Here's how the part is built. I have some questions about the finished solid (model axes, mm). A direction names the side the tool comes from. Give positions to 0.01 mm unless a question says otherwise; leave off trailing zeros. Loops run counter-clockwise (first coordinate to the right, second up) from the corner with the lowest first, then second, coordinate; pieces in that order, holes last.
Q1. I need wall thicknesses on probe 1 along Y at (x, z) = (26.5, 4.1); probe 2 along Z at (x, y) = (-17.5, -10.25). Which ranges of each line are inside material? Lowest first, please.
Q2. Suppose I cut it at A-A (x = 2.5). List the corners of the cut face in (y, z) for me.
Q3. For faces 1 (the face through (0, 10, 4)), 2 (the face through (0, -11, 2.5)), 3 (the face through (-30, 0, 2)), which set-ups out of +Z, -Z, +X, -X, +Y, -Y let a thin tool reach every point of the face, with its end or its side?
Q4. Suppose I cut it at B-B (z = 4.25). List the corners of the cut face in (x, y) for me, and give its area (3 significant figures).
Q5. I'm going to push flat-ended pins straight in: P1, Ø2, axis at x = 14, y = -11.5, coming from the +Z side; P2, Ø1.5, axis at x = 0, y = 7.5, coming from the -Z side; P3, Ø0.8, axis at x = -3.5, z = 3.5, coming from the +Y side; P4, Ø2, axis at x = 2, z = 4, coming from the -Y side. Where does each tip first touch, or does it pass through?
```python
from build123d import *

# Parameters (mm, degrees)
SKETCH_1_W      = 60
SKETCH_1_H      = 25
EXTRUDE_1_DEPTH = 2.5
SKETCH_2_W      = 60
SKETCH_2_H      = 20
EXTRUDE_2_DEPTH = 2.5


with BuildPart() as part:
    # Эскиз1 → Бобышка-Вытянуть1 (new body)
    with BuildSketch(Plane.XY):
        Rectangle(SKETCH_1_W, SKETCH_1_H)
    extrude(amount=EXTRUDE_1_DEPTH)

    # Эскиз2 → Бобышка-Вытянуть2 (add)
    with BuildSketch(Plane.XY.offset(2.5)):
        Rectangle(SKETCH_2_W, SKETCH_2_H)
    extrude(amount=EXTRUDE_2_DEPTH)


solid = part.part
```
Solutions:
1. probe 1: y = -10 to 10
1. probe 2: z = 0 to 2.5
2. outline: (-12.5, 0) - (12.5, 0) - (12.5, 2.5) - (10, 2.5) - (10, 5) - (-10, 5) - (-10, 2.5) - (-12.5, 2.5) - close
3. face 1: +Z, +X, -X, +Y
3. face 2: +Z, +X, -X, -Y
3. face 3: +Z, -Z, -X, +Y, -Y
4. outline: (-30, -10) - (30, -10) - (30, 10) - (-30, 10) - close
4. area: 1,200 mm2
5. P1: stops at z = 2.5
5. P2: stops at z = 0
5. P3: stops at y = 10
5. P4: stops at y = -10
